Read the model definition and answer for the solid it produces. Units are mm, in the model's axes. Face numbers are marked on the shaded views. A direction names the side the tool comes from. Coordinates: 2 decimals unless noted, no trailing zeros.
(1) Find the intervals of material crossed by probe 1 along Y at (x, z) = (-12, 11.5); probe 2 along Z at (x, y) = (-7, 6.25); probe 3 along X at (y, z) = (6.75, -13), in increasing order.
(2) Given pin 1 (6 mm diameter, centred on y = 2, z = 3, fed in from -X); pin 2 (1.5 mm diameter, centred on y = 0, z = -1.5, fed in from -X); pin 3 (1 mm diameter, centred on x = 2, y = -2, fed in from +Z), each flat-ended and moving along its own axis, determine where each tip first touches the part or whether it passes through.
(3) The mould has two halves that part along Z. Classify the marked faces 1, 2, 3 and 4: +Z half, -Z half, draft (parallel to the pull), parting line (faces both ways), or undercut.
(4) Which of the six approach directions +Z, -Z, +X, -X, +Y, -Y give full straight-line access (tool end or side, diameter ignored) to the marked faces 5, 6 and 7?
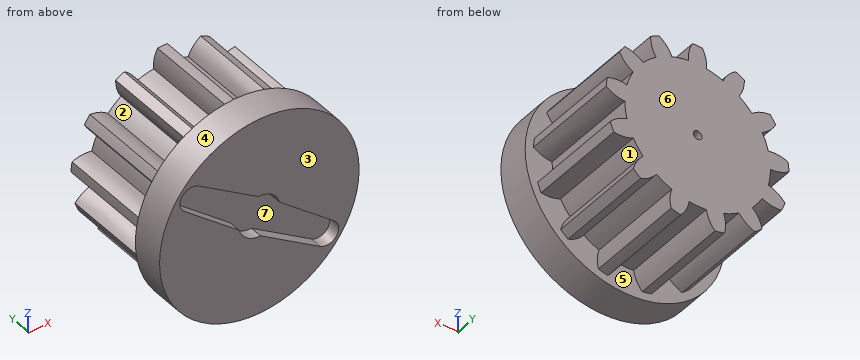
from build123d import *
from OCP.BRepAlgoAPI import BRepAlgoAPI_Cut
from OCP.TopTools import TopTools_ListOfShape

# Parameters (mm, degrees)
SKETCH1_R           = 0.4
BOSS_EXTRUDE1_DEPTH = 9
SKETCH2_R           = 9.25
BOSS_EXTRUDE2_DEPTH = 3
SCALE1_SCALE        = 1.8
CUT_EXTRUDE1_DEPTH  = 2


with BuildPart() as part:
    # Sketch1 → Boss-Extrude1 (new body)
    with BuildSketch(Plane(origin=(0, 0, 0), x_dir=(1, 0, 0), z_dir=(0, 1, 0))):
        with BuildLine():
            add(Edge.make_bspline(
                [(-5.065227978, 4.461610195), (-5.526615005, 4.86619147), (-5.830003112, 5.39406146), (-5.975392301, 6.045220165)],
                knots=[0, 0, 0, 0, 0.872429449, 0.872429449, 0.872429449, 0.872429449], degree=3))
            ThreePointArc((-5.065227978, 4.461610195), (-5.560258819, 3.827012132), (-5.976238464, 3.138004752))
            add(Edge.make_bspline(
                [(-7.780961116, 3.42149735), (-7.125870497, 3.507536778), (-6.52429628, 3.413039245), (-5.976238464, 3.138004752)],
                knots=[0.127683247, 0.127683247, 0.127683247, 0.127683247, 1, 1, 1, 1], degree=3))
            ThreePointArc((-7.780961116, 3.42149735), (-7.951879756, 3.00293329), (-8.10030101, 2.575873357))
            add(Edge.make_bspline(
                [(-6.558450277, 1.596630818), (-7.155006493, 1.740452504), (-7.668956737, 2.066866683), (-8.10030101, 2.575873357)],
                knots=[0, 0, 0, 0, 0.872429449, 0.872429449, 0.872429449, 0.872429449], degree=3))
            ThreePointArc((-6.558450277, 1.596630818), (-6.701865893, 0.804669837), (-6.749999881, 0.00126872))
            add(Edge.make_bspline(
                [(-8.479748007, -0.586407486), (-7.939678588, -0.205787566), (-7.363095879, -0.009895497), (-6.749999881, 0.00126872)],
                knots=[0.127683247, 0.127683247, 0.127683247, 0.127683247, 1, 1, 1, 1], degree=3))
            ThreePointArc((-8.479748007, -0.586407486), (-8.436572529, -1.036457408), (-8.369528376, -1.483574994))
            add(Edge.make_bspline(
                [(-6.549210655, -1.634117437), (-7.144272221, -1.784003157), (-7.751044795, -1.733822342), (-8.369528376, -1.483574994)],
                knots=[0, 0, 0, 0, 0.872429449, 0.872429449, 0.872429449, 0.872429449], degree=3))
            ThreePointArc((-6.549210655, -1.634117437), (-6.308156258, -2.402012621), (-5.977417671, -3.13575796))
            add(Edge.make_bspline(
                [(-7.235926822, -4.459973434), (-6.934601997, -3.871968458), (-6.515098947, -3.4305633), (-5.977417671, -3.13575796)],
                knots=[0.127683247, 0.127683247, 0.127683247, 0.127683247, 1, 1, 1, 1], degree=3))
            ThreePointArc((-7.235926822, -4.459973434), (-6.988548208, -4.838408204), (-6.721397655, -5.203154193))
            add(Edge.make_bspline(
                [(-5.039625799, -4.490509081), (-5.496871281, -4.899765193), (-6.0574619, -5.137313564), (-6.721397655, -5.203154193)],
                knots=[0, 0, 0, 0, 0.872429449, 0.872429449, 0.872429449, 0.872429449], degree=3))
            ThreePointArc((-5.039625799, -4.490509081), (-4.469324045, -5.058422935), (-3.835481109, -5.554420281))
            add(Edge.make_bspline(
                [(-4.334442004, -7.311813216), (-4.34089166, -6.651128039), (-4.174571361, -6.065330394), (-3.835481109, -5.554420281)],
                knots=[0.127683247, 0.127683247, 0.127683247, 0.127683247, 1, 1, 1, 1], degree=3))
            ThreePointArc((-4.334442004, -7.311813216), (-3.939531713, -7.53193799), (-3.533475733, -7.730753472))
            add(Edge.make_bspline(
                [(-2.375523406, -6.318179211), (-2.590203375, -6.893050073), (-2.976187484, -7.36390816), (-3.533475733, -7.730753472)],
                knots=[0, 0, 0, 0, 0.872429449, 0.872429449, 0.872429449, 0.872429449], degree=3))
            ThreePointArc((-2.375523406, -6.318179211), (-1.606623554, -6.556009515), (-0.814882047, -6.700631854))
            add(Edge.make_bspline(
                [(-0.439988759, -8.488604708), (-0.752735357, -7.906594341), (-0.877699786, -7.31060339), (-0.814882047, -6.700631854)],
                knots=[0.127683247, 0.127683247, 0.127683247, 0.127683247, 1, 1, 1, 1], degree=3))
            ThreePointArc((-0.439988759, -8.488604708), (0.011984021, -8.499991552), (0.463922896, -8.487330296))
            add(Edge.make_bspline(
                [(0.832782771, -6.698430626), (0.909848909, -7.307220251), (0.786895617, -7.903520141), (0.463922896, -8.487330296)],
                knots=[0, 0, 0, 0, 0.872429449, 0.872429449, 0.872429449, 0.872429449], degree=3))
            ThreePointArc((0.832782771, -6.698430626), (1.624135031, -6.551693323), (2.392396671, -6.311809421))
            add(Edge.make_bspline(
                [(3.555260608, -7.72075916), (3.007863545, -7.350755165), (2.620242233, -6.881105252), (2.392396671, -6.311809421)],
                knots=[0.127683247, 0.127683247, 0.127683247, 0.127683247, 1, 1, 1, 1], degree=3))
            ThreePointArc((3.555260608, -7.72075916), (3.96075436, -7.520799485), (4.355042381, -7.299562032))
            add(Edge.make_bspline(
                [(3.850308451, -5.54415231), (4.201465773, -6.047394331), (4.369710416, -6.632530905), (4.355042381, -7.299562032)],
                knots=[0, 0, 0, 0, 0.872429449, 0.872429449, 0.872429449, 0.872429449], degree=3))
            ThreePointArc((3.850308451, -5.54415231), (4.482823853, -5.046463148), (5.051606144, -4.477027515))
            add(Edge.make_bspline(
                [(6.736042616, -5.184180734), (6.079397157, -5.110946566), (5.517918333, -4.875228826), (5.051606144, -4.477027515)],
                knots=[0.127683247, 0.127683247, 0.127683247, 0.127683247, 1, 1, 1, 1], degree=3))
            ThreePointArc((6.736042616, -5.184180734), (7.002163607, -4.818682892), (7.24847414, -4.439552076))
            add(Edge.make_bspline(
                [(5.985774866, -3.119775513), (6.530577461, -3.402183249), (6.951477219, -3.84210877), (7.24847414, -4.439552076)],
                knots=[0, 0, 0, 0, 0.872429449, 0.872429449, 0.872429449, 0.872429449], degree=3))
            ThreePointArc((5.985774866, -3.119775513), (6.314551754, -2.385149082), (6.553553527, -1.616612559))
            add(Edge.make_bspline(
                [(8.373678438, -1.459968977), (7.758214146, -1.700281702), (7.151505842, -1.75249623), (6.553553527, -1.616612559)],
                knots=[0.127683247, 0.127683247, 0.127683247, 0.127683247, 1, 1, 1, 1], degree=3))
            ThreePointArc((8.373678438, -1.459968977), (8.439461558, -1.01266412), (8.481367828, -0.562494242))
            add(Edge.make_bspline(
                [(6.749972396, 0.019304256), (7.363612555, 0.022427015), (7.940744366, -0.171505818), (8.481367828, -0.562494242)],
                knots=[0, 0, 0, 0, 0.872429449, 0.872429449, 0.872429449, 0.872429449], degree=3))
            ThreePointArc((6.749972396, 0.019304256), (6.699691947, 0.822573894), (6.554160776, 1.614148852))
            add(Edge.make_bspline(
                [(8.093005444, 2.598704077), (7.65971777, 2.099897208), (7.146769547, 1.771712133), (6.554160776, 1.614148852)],
                knots=[0.127683247, 0.127683247, 0.127683247, 0.127683247, 1, 1, 1, 1], degree=3))
            ThreePointArc((8.093005444, 2.598704077), (7.943380571, 3.025343799), (7.771282357, 3.443424244))
            add(Edge.make_bspline(
                [(5.967832596, 3.153961653), (6.509732754, 3.44189952), (7.110882674, 3.53838705), (7.771282357, 3.443424244)],
                knots=[0, 0, 0, 0, 0.872429449, 0.872429449, 0.872429449, 0.872429449], degree=3))
            ThreePointArc((5.967832596, 3.153961653), (5.550013455, 3.841855105), (5.053288778, 4.475128213))
            add(Edge.make_bspline(
                [(5.958322434, 6.062045345), (5.806472362, 5.419014975), (5.504794477, 4.890042598), (5.053288778, 4.475128213)],
                knots=[0.127683247, 0.127683247, 0.127683247, 0.127683247, 1, 1, 1, 1], degree=3))
            ThreePointArc((5.958322434, 6.062045345), (5.627566824, 6.370281912), (5.280889753, 6.660495734))
            add(Edge.make_bspline(
                [(3.818534268, 5.566084444), (4.16455163, 6.072874324), (4.652003458, 6.437678087), (5.280889753, 6.660495734)],
                knots=[0, 0, 0, 0, 0.872429449, 0.872429449, 0.872429449, 0.872429449], degree=3))
            ThreePointArc((3.818534268, 5.566084444), (3.128893766, 5.98101361), (2.394769219, 6.310909632))
            add(Edge.make_bspline(
                [(2.45865956, 8.136645081), (2.623034112, 7.496701718), (2.601737332, 6.888123235), (2.394769219, 6.310909632)],
                knots=[0.127683247, 0.127683247, 0.127683247, 0.127683247, 1, 1, 1, 1], degree=3))
            ThreePointArc((2.45865956, 8.136645081), (2.022545337, 8.25586521), (1.580708948, 8.351727918))
            add(Edge.make_bspline(
                [(0.794455758, 6.703084368), (0.865321915, 7.312626807), (1.127406312, 7.862174657), (1.580708948, 8.351727918)],
                knots=[0, 0, 0, 0, 0.872429449, 0.872429449, 0.872429449, 0.872429449], degree=3))
            ThreePointArc((0.794455758, 6.703084368), (-0.009017778, 6.749993976), (-0.812363108, 6.700937709))
            add(Edge.make_bspline(
                [(-1.604252589, 8.347237485), (-1.161309642, 7.856984441), (-0.897346481, 7.308217849), (-0.812363108, 6.700937709)],
                knots=[0.127683247, 0.127683247, 0.127683247, 0.127683247, 1, 1, 1, 1], degree=3))
            ThreePointArc((-1.604252589, 8.347237485), (-2.045816912, 8.250129282), (-2.481593228, 8.129679886))
            add(Edge.make_bspline(
                [(-2.411622992, 6.304488444), (-2.632142622, 6.877144615), (-2.655466033, 7.485541762), (-2.481593228, 8.129679886)],
                knots=[0, 0, 0, 0, 0.872429449, 0.872429449, 0.872429449, 0.872429449], degree=3))
            ThreePointArc((-2.411622992, 6.304488444), (-3.144863458, 5.972632069), (-3.833392837, 5.555861712))
            add(Edge.make_bspline(
                [(-5.299649804, 6.645578377), (-4.679611352, 6.417326717), (-4.19085903, 6.054087828), (-3.833392837, 5.555861712)],
                knots=[0.127683247, 0.127683247, 0.127683247, 0.127683247, 1, 1, 1, 1], degree=3))
            ThreePointArc((-5.299649804, 6.645578377), (-5.645507162, 6.35438816), (-5.975392301, 6.045220165))
        make_face()
        with Locations(Location((0, 0, 0), (0, 0, 270))):
            Circle(SKETCH1_R, mode=Mode.SUBTRACT)
    extrude(amount=BOSS_EXTRUDE1_DEPTH)

    # Sketch2 → Boss-Extrude2 (add)
    with BuildSketch(Plane.XZ):
        with Locations(Location((0, 0, 0), (0, 0, 270))):
            Circle(SKETCH2_R)
    extrude(amount=BOSS_EXTRUDE2_DEPTH)


with BuildPart() as part_1:
    # Scale1: scaled about (0, 2.477742253, 0)
    add(part.part.scale(SCALE1_SCALE).moved(Location((0, -1.982193802, 0))))


with BuildPart() as cut_extrude1_tool:
    # Sketch3 → Cut-Extrude1 (new body)
    with BuildSketch(Plane.XZ.offset(7.382189851)):
        with BuildLine():
            Line((-10.14806543, 10.074005921), (-0.183742843, 3.445103564))
            ThreePointArc((-0.183742843, 3.445103564), (2.064801156, 2.763891493), (3.355756213, 0.800874672))
            Line((3.355756213, 0.800874672), (12.53847182, -6.874267357))
            ThreePointArc((12.53847182, -6.874267357), (12.858103903, -9.605814074), (10.14806543, -10.074005921))
            Line((10.14806543, -10.074005921), (0.183742843, -3.445103564))
            ThreePointArc((0.183742843, -3.445103564), (-2.064801156, -2.763891493), (-3.355756213, -0.800874672))
            Line((-3.355756213, -0.800874672), (-12.53847182, 6.874267357))
            ThreePointArc((-12.53847182, 6.874267357), (-12.858103903, 9.605814074), (-10.14806543, 10.074005921))
        make_face()
    extrude(amount=-CUT_EXTRUDE1_DEPTH)


with BuildPart() as part_2:
    add(part_1.part)

    # Cut-Extrude1: cut by cut_extrude1_tool, with a tolerance
    cut_extrude1_stock = TopTools_ListOfShape()
    cut_extrude1_stock.Append(part_2.part.wrapped)
    cut_extrude1_tools = TopTools_ListOfShape()
    cut_extrude1_tools.Append(cut_extrude1_tool.part.wrapped)
    cut_extrude1_cut = BRepAlgoAPI_Cut()
    cut_extrude1_cut.SetArguments(cut_extrude1_stock)
    cut_extrude1_cut.SetTools(cut_extrude1_tools)
    cut_extrude1_cut.SetFuzzyValue(0.00001)
    cut_extrude1_cut.Build()
    add(Compound.cast(cut_extrude1_cut.Shape()).solids(), mode=Mode.REPLACE)


solid = part_2.part
Response:
1. probe 1: y = -7.38 to -1.98
1. probe 2: z = -10.14 to 9.93, 10.15 to 13.6
1. probe 3: x = -4.67 to -1.68, 1.63 to 4.62
2. pin 1: stops at x = -15.26
2. pin 2: stops at x = -12.13
2. pin 3: stops at z = 16.58
3. face 1: undercut
3. face 2: undercut
3. face 3: draft
3. face 4: parting line
4. face 5: +Y
4. face 6: +Z, -Z, +X, -X, +Y
4. face 7: -Y
